from build123d import *

# Parameters (mm, degrees)
SKETCH1_W            = 539
SKETCH1_H            = 299
BOSS_EXTRUDE1_DEPTH  = 12
SKETCH15_W           = 70
SKETCH15_H           = 20
CUT_EXTRUDE8_DEPTH   = 309.422599691
SKETCH2_W            = 30
SKETCH2_H            = 51
CUT_EXTRUDE1_DEPTH   = 309.422599691
SKETCH4_W            = 229
SKETCH4_H            = 168
CUT_EXTRUDE2_DEPTH   = 3.75
SKETCH5_W            = 18
SKETCH5_H            = 299
CUT_EXTRUDE3_DEPTH   = 4.25
SKETCH6_W            = 11
SKETCH6_H            = 49.5
CUT_EXTRUDE4_DEPTH   = 1.75
SKETCH7_W            = 17
SKETCH7_H            = 168
BOSS_EXTRUDE3_DEPTH  = 1.7
M6_CLEARANCE_HOLE1_D = 6.6
SKETCH10_W           = 18
SKETCH10_H           = 28.8
BOSS_EXTRUDE4_DEPTH  = 4.25
CUT_EXTRUDE5_DEPTH   = 1.5
SKETCH13_W           = 20
SKETCH13_H           = 1.5
CUT_EXTRUDE6_DEPTH   = 5.25
SKETCH14_W           = 20
SKETCH14_H           = 64
CUT_EXTRUDE7_DEPTH   = 1.5


with BuildPart() as part:
    # Sketch1 → Boss-Extrude1 (new body)
    with BuildSketch(Plane(origin=(0, 0, 0), x_dir=(1, 0, 0), z_dir=(0, 1, 0))):
        Rectangle(SKETCH1_W, SKETCH1_H)
    extrude(amount=-BOSS_EXTRUDE1_DEPTH)

    # Sketch15 → Cut-Extrude8 (cut, through all)
    with BuildSketch(Plane(origin=(0, 0, 0), x_dir=(1, 0, 0), z_dir=(0, 1, 0))):
        Polygon((269.5, 149.5), (199.5, 149.5), (199.5, 129.5), (249.5, 129.5), (249.5, 91.5), (269.5, 91.5), align=None)
        with Locations((234.5, -139.5)):
            Rectangle(SKETCH15_W, SKETCH15_H)
    extrude(amount=-CUT_EXTRUDE8_DEPTH, mode=Mode.SUBTRACT)

    # Sketch2 → Cut-Extrude1 (cut, through all)
    with BuildSketch(Plane(origin=(0, 0, 0), x_dir=(1, 0, 0), z_dir=(0, 1, 0))):
        with Locations((-254.5, 0)):
            Rectangle(SKETCH2_W, SKETCH2_H)
    cut_extrude1 = extrude(amount=-CUT_EXTRUDE1_DEPTH, mode=Mode.SUBTRACT)

    # Mirror1: Cut-Extrude1 across plane
    add(cut_extrude1.mirror(Plane(origin=(0, 0, 0), x_dir=(0, 0, 1), z_dir=(1, 0, 0))), mode=Mode.SUBTRACT)

    # Sketch4 → Cut-Extrude2 (cut)
    with BuildSketch(Plane(origin=(0, 0, 0), x_dir=(1, 0, 0), z_dir=(0, 1, 0))):
        with Locations((14, 0)):
            Rectangle(SKETCH4_W, SKETCH4_H)
    extrude(amount=-CUT_EXTRUDE2_DEPTH, mode=Mode.SUBTRACT)

    # Sketch5 → Cut-Extrude3 (cut)
    with BuildSketch(Plane(origin=(0, 0, 0), x_dir=(1, 0, 0), z_dir=(0, 1, 0))):
        with Locations((-120.5, 0)):
            Rectangle(SKETCH5_W, SKETCH5_H)
    extrude(amount=-CUT_EXTRUDE3_DEPTH, mode=Mode.SUBTRACT)

    # Sketch6 → Cut-Extrude4 (cut)
    with BuildSketch(Plane(origin=(0, 0, 0), x_dir=(1, 0, 0), z_dir=(0, 1, 0))):
        with Locations((-106, 39.15)):
            Rectangle(SKETCH6_W, SKETCH6_H)
        with Locations((-106, -39.15)):
            Rectangle(SKETCH6_W, SKETCH6_H)
    extrude(amount=-CUT_EXTRUDE4_DEPTH, mode=Mode.SUBTRACT)

    # Sketch7 → Boss-Extrude3 (add)
    with BuildSketch(Plane(origin=(0, -3.75, 0), x_dir=(1, 0, 0), z_dir=(0, 1, 0))):
        with Locations((-92, 0)):
            Rectangle(SKETCH7_W, SKETCH7_H)
    extrude(amount=BOSS_EXTRUDE3_DEPTH)

    # M6 Clearance Hole1 (through all)
    with Locations(Plane(origin=(-255, -12, 105), x_dir=(0, 0, -1), z_dir=(0, -1, 0))):
        with Locations((0, 0), (70, 0), (210, 0), (140, 0), (210, 85), (140, 85), (70, 85), (0, 85), (0, 255), (0, 340), (0, 425), (0, 510), (70, 510), (70, 425), (70, 340), (70, 255), (70, 170), (140, 170), (140, 255), (140, 340), (140, 425), (140, 510), (210, 425), (210, 340), (210, 255), (210, 170)):
            Hole(M6_CLEARANCE_HOLE1_D / 2)

    # Sketch10 → Boss-Extrude4 (add)
    with BuildSketch(Plane(origin=(0, -4.25, 0), x_dir=(1, 0, 0), z_dir=(0, 1, 0))):
        with Locations((-120.5, 0)):
            Rectangle(SKETCH10_W, SKETCH10_H)
    extrude(amount=BOSS_EXTRUDE4_DEPTH)

    # Sketch12 → Cut-Extrude5 (cut)
    with BuildSketch(Plane(origin=(0, -3.75, 0), x_dir=(1, 0, 0), z_dir=(0, 1, 0))):
        Polygon((32.5, -10), (32.5, -84), (12.5, -84), (12.5, -10), (-20.5, -10), (-20.5, -84), (-40.5, -84), (-40.5, -10), (-63.5, -10), (-63.5, -84), (-83.5, -84), (-83.5, 84), (-63.5, 84), (-63.5, 10), (-40.5, 10), (-40.5, 84), (-20.5, 84), (-20.5, 10), (12.5, 10), (12.5, 84), (32.5, 84), (32.5, 10), (65.5, 10), (65.5, 84), (85.5, 84), (85.5, 10), (108.5, 10), (108.5, 84), (128.5, 84), (128.5, -84), (108.5, -84), (108.5, -10), (85.5, -10), (85.5, -84), (65.5, -84), (65.5, -10), align=None)
    extrude(amount=-CUT_EXTRUDE5_DEPTH, mode=Mode.SUBTRACT)

    # Sketch13 → Cut-Extrude6 (cut)
    with BuildSketch(Plane(origin=(0, 0, 0), x_dir=(1, 0, 0), z_dir=(0, 1, 0))):
        with Locations((-73.5, -84.75)):
            Rectangle(SKETCH13_W, SKETCH13_H)
        with Locations((-30.5, -84.75)):
            Rectangle(SKETCH13_W, SKETCH13_H)
        with Locations((22.5, -84.75)):
            Rectangle(SKETCH13_W, SKETCH13_H)
        with Locations((75.5, -84.75)):
            Rectangle(SKETCH13_W, SKETCH13_H)
        with Locations((118.5, -84.75)):
            Rectangle(SKETCH13_W, SKETCH13_H)
    extrude(amount=-CUT_EXTRUDE6_DEPTH, mode=Mode.SUBTRACT)

    # Sketch14 → Cut-Extrude7 (cut)
    with BuildSketch(Plane(origin=(0, 0, 0), x_dir=(1, 0, 0), z_dir=(0, 1, 0))):
        with Locations((-73.5, -117.5)):
            Rectangle(SKETCH14_W, SKETCH14_H)
        with Locations((-30.5, -117.5)):
            Rectangle(SKETCH14_W, SKETCH14_H)
        with Locations((22.5, -117.5)):
            Rectangle(SKETCH14_W, SKETCH14_H)
        with Locations((75.5, -117.5)):
            Rectangle(SKETCH14_W, SKETCH14_H)
        with Locations((118.5, -117.5)):
            Rectangle(SKETCH14_W, SKETCH14_H)
    extrude(amount=-CUT_EXTRUDE7_DEPTH, mode=Mode.SUBTRACT)


solid = part.part
Can you work these out from the model? Positions are in its coordinate system, mm. A direction names the side the tool comes from. Give positions to 0.01 mm unless a question says otherwise; leave off trailing zeros. Use one line per item in the form item = value.
Item 1: Will these pins go through, and if not, where does the flat tip stop? pin 1 Ø6 at (y, z) = (-9, -6.5) entering from -X; pin 2 Ø6 at (x, z) = (47, 48.5) entering from +Y; pin 3 Ø12 at (x, z) = (-83.5, 18.5) entering from +Y.
Values follow:
pin_1 = -239.5
pin_2 = -3.75
pin_3 = -2.05
Item 2: If we section it at B-B, the plane y = -9.75: Count the separate pieces of the cut face and the enclosed holes in it, and give its area (3 significant figures).
Values follow:
separate_pieces = 1
enclosed_holes = 26
area = 154,000 mm^2
Item 3: If I drill on line 1 along Z through (x, y) = (-255, -3.75); line 2 along Z through (x, y) = (-170, -7.5); line 3 along X through (y, z) = (-2.5, 129), over which ranges is the centre line in solid material (lowest first)? Write a range as [from, to].
Values follow:
line_1 = [-149.5, -108.3], [-101.7, -38.3], [-31.7, -25.5], [25.5, 31.7], [38.3, 101.7], [108.3, 149.5]
line_2 = [-149.5, -108.3], [-101.7, -38.3], [-31.7, 31.7], [38.3, 101.7], [108.3, 149.5]
line_3 = [-269.5, -129.5], [-111.5, 269.5]
Item 4: Thinking about a two-plate mould opening in Z: for faces 4 (the flat face through (49, 0, 116)), 5 (the flat face through (-255, -6, 25.5)), 6 (the flat face through (-38, -6, 149.5)), which applies, pulls with the +Z half, pulls with the -Z half, needs draft (parallel to the pull), parting line crosses it, or undercut?
Values follow:
face_4 = needs draft
face_5 = undercut
face_6 = pulls with the +Z half
Item 5: For faces 1 (the flat face through (255, -6, -25.5)), 2 (the flat face through (49, -3.75, -48)), 3 (the flat face through (-121, -4.25, 81)), which set-ups out of +Z, -Z, +X, -X, +Y, -Y let a thin tool reach every point of the face, with its end or its side?
Values follow:
face_1 = +X, +Y, -Y
face_2 = +Y
face_3 = +Z, +Y
